from build123d import *

# Parameters (mm, degrees)
SKETCH1_W               = 50
SKETCH1_H               = 70
BOSS_EXTRUDE1_DEPTH     = 2
SKETCH2_R               = 5
SKETCH2_R_2             = 2.5
BOSS_EXTRUDE2_DEPTH     = 70
SKETCH3_R               = 2.5
CUT_EXTRUDE1_DEPTH      = 47.786750261
CUT_EXTRUDE2_DEPTH      = 47.786750261
CUT_EXTRUDE2_DEPTH_BACK = 47.786750261
SKETCH4_W               = 10
SKETCH4_H               = 14


with BuildPart() as part:
    # Sketch1 → Boss-Extrude1 (new body)
    with BuildSketch(Plane(origin=(0, 0, 0), x_dir=(1, 0, 0), z_dir=(0, 1, 0))):
        Rectangle(SKETCH1_W, SKETCH1_H)
    extrude(amount=BOSS_EXTRUDE1_DEPTH)

    # Sketch2 → Boss-Extrude2 (add)
    with BuildSketch(Plane.XY.offset(35)):
        with Locations((-25, 5)):
            Circle(SKETCH2_R)
        with Locations((-25, 5)):
            Circle(SKETCH2_R_2, mode=Mode.SUBTRACT)
    extrude(amount=-BOSS_EXTRUDE2_DEPTH)

    # Sketch3 → Cut-Extrude1 (cut, through all)
    with BuildSketch(Plane(origin=(0, 2, 0), x_dir=(1, 0, 0), z_dir=(0, 1, 0))):
        with Locations(Location((0, 15, 0), (0, 0, 270))):
            Circle(SKETCH3_R)
        with Locations(Location((0, -15, 0), (0, 0, 270))):
            Circle(SKETCH3_R)
    extrude(amount=-CUT_EXTRUDE1_DEPTH, mode=Mode.SUBTRACT)

    # Sketch4 → Cut-Extrude2 (cut, two sides: drawn at the far end of the back side and taken through both)
    with BuildSketch(Plane(origin=(0, 2, 0), x_dir=(1, 0, 0), z_dir=(0, 1, 0)).offset(-CUT_EXTRUDE2_DEPTH_BACK)):
        with Locations((-25, 28)):
            Rectangle(SKETCH4_W, SKETCH4_H)
        with Locations((-25, 0.360390559)):
            Rectangle(SKETCH4_W, SKETCH4_H)
        with Locations((-25, -28)):
            Rectangle(SKETCH4_W, SKETCH4_H)
    extrude(amount=CUT_EXTRUDE2_DEPTH + CUT_EXTRUDE2_DEPTH_BACK, mode=Mode.SUBTRACT)


solid = part.part
Could you check a few things on this model? Use its own coordinates, in mm. A direction names the side the tool comes from. Coordinates: 2 decimals unless noted, no trailing zeros. Loops run counter-clockwise (first coordinate to the right, second up) from the corner with the lowest first, then second, coordinate; pieces in that order, holes last.
1. For faces 1 (the face through (-23, 3, 6.64)), 2 (the face through (-23, 3, 21)), 3 (the face through (-23, 3, -21)), which set-ups out of +Z, -Z, +X, -X, +Y, -Y let a thin tool reach every point of the face, with its end or its side?
2. For P1, Ø5, axis at x = -23.5, y = 6, coming from the +Z side; P2, Ø1, axis at y = 0.5, z = 2.5, coming from the -X side; P3, Ø6, axis at x = 19.5, y = 6.5, coming from the -Z side; P4, Ø6, axis at x = -25, y = 5, coming from the -Z side, each with a flat end and sliding along its axis, tell me the tip position at first contact or that it passes through.
3. Imagine slicing it at B-B (y = 5). Please give me the cut outline in (x, z).
4. Imagine slicing it at C-C (x = 0). Please give me the cut outline in (y, z), and give its area (3 significant figures).
5. Imagine slicing it at A-A (z = 15). Please give me the cut outline in (x, y).
6. Imagine slicing it at D-D (z = -10). Please give me the cut outline in (x, y).
7. We'd pull the mould along X, two halves only. Please class faces 4 (the face through (0.1, 1, -17.5)), 5 (the face through (-20, 1, -28)), 6 (the face through (-26.84, 6.69, -14.08)), 7 (the face through (-23, 3, -7.36)): released by +X, released by -X, zero draft, split by the parting line, or undercut.
8. I need wall thicknesses on L1, parallel to Y at x = -25, z = 16; L2, parallel to Z at x = -20.5, y = 1.25; L3, parallel to Y at x = 6, z = 20.5. Which ranges of each line are inside material? Lowest first, please.
Computed values:
1. face 1: -X, +Y, -Y
1. face 2: +Z, -X, +Y, -Y
1. face 3: -Z, -X, +Y, -Y
2. P1: stops at z = 21
2. P2: stops at x = -20
2. P3: passes through
2. P4: stops at z = -21
3. outline: (-30, -21) - (-27.5, -21) - (-27.5, -7.36) - (-30, -7.36) - close; (-30, 6.64) - (-27.5, 6.64) - (-27.5, 21) - (-30, 21) - close; (-22.5, -21) - (-20, -21) - (-20, -7.36) - (-22.5, -7.36) - close; (-22.5, 6.64) - (-20, 6.64) - (-20, 21) - (-22.5, 21) - close
4. outline: (0, -35) - (2, -35) - (2, -17.5) - (0, -17.5) - close; (0, -12.5) - (2, -12.5) - (2, 12.5) - (0, 12.5) - close; (0, 17.5) - (2, 17.5) - (2, 35) - (0, 35) - close
4. area: 120 mm2
5. outline: (-25, 0) - (-2.5, 0) - (-2.5, 2) - (-21, 2) arc R5 ccw (long way) to start; (2.5, 0) - (25, 0) - (25, 2) - (2.5, 2) - close; hole circle Ø5 at (-25, 5)
6. outline: (-25, 0) - (25, 0) - (25, 2) - (-21, 2) arc R5 ccw (long way) to start; hole circle Ø5 at (-25, 5)
7. face 4: undercut
7. face 5: released by -X
7. face 6: undercut
7. face 7: zero draft
8. L1: y = 0 to 2.5, 7.5 to 10
8. L2: z = -21 to -7.36, 6.64 to 21
8. L3: y = 0 to 2
